Geometry check sheet. Reference: the model listing, model coordinates, mm. Give positions to 0.01 mm unless a question says otherwise; leave off trailing zeros.
```python
from build123d import *

# Parameters (mm, degrees)
SKETCH_1_R          = 2.5
EXTRUDE_1_DEPTH     = 506.79
CUT_EXTRUDE_1_DEPTH = 508.341254196


with BuildPart() as part:
    # 草图1 → 凸台-拉伸1 (new body)
    with BuildSketch(Plane(origin=(0, 0, 0), x_dir=(1, 0, 0), z_dir=(0, 1, 0))):
        with BuildLine():
            Line((-10.811269129, -4.789644731), (-12.611269129, -4.789644731))
            Line((-12.611269129, -4.789644731), (-12.611269129, -10.189644731))
            ThreePointArc((-12.611269129, -10.189644731), (-12.171929301, -11.250304902), (-11.111269129, -11.689644731))
            Line((-11.111269129, -11.689644731), (-5.711269129, -11.689644731))
            Line((-5.711269129, -11.689644731), (-5.711269129, -9.889644731))
            Line((-5.711269129, -9.889644731), (-8.111269129, -9.889644731))
            Line((-8.111269129, -9.889644731), (-8.111269129, -8.086694886))
            Line((-8.111269129, -8.086694886), (-4.814218974, -4.789644731))
            Line((-4.814218974, -4.789644731), (-0.408319284, -4.789644731))
            Line((-0.408319284, -4.789644731), (2.888730871, -8.086694886))
            Line((2.888730871, -8.086694886), (2.888730871, -9.889644731))
            Line((2.888730871, -9.889644731), (0.488730871, -9.889644731))
            Line((0.488730871, -9.889644731), (0.488730871, -11.689644731))
            Line((0.488730871, -11.689644731), (5.888730871, -11.689644731))
            ThreePointArc((5.888730871, -11.689644731), (6.949391043, -11.250304902), (7.388730871, -10.189644731))
            Line((7.388730871, -10.189644731), (7.388730871, -4.789644731))
            Line((7.388730871, -4.789644731), (5.588730871, -4.789644731))
            Line((5.588730871, -4.789644731), (5.588730871, -7.189644731))
            Line((5.588730871, -7.189644731), (3.785781026, -7.189644731))
            Line((3.785781026, -7.189644731), (0.442857891, -3.846721596))
            Line((0.442857891, -3.846721596), (0.442857891, 0.467432135))
            Line((0.442857891, 0.467432135), (3.785781026, 3.810355269))
            Line((3.785781026, 3.810355269), (5.588730871, 3.810355269))
            Line((5.588730871, 3.810355269), (5.588730871, 1.410355269))
            Line((5.588730871, 1.410355269), (7.388730871, 1.410355269))
            Line((7.388730871, 1.410355269), (7.388730871, 6.810355269))
            ThreePointArc((7.388730871, 6.810355269), (6.949391043, 7.871015441), (5.888730871, 8.310355269))
            Line((5.888730871, 8.310355269), (0.488730871, 8.310355269))
            Line((0.488730871, 8.310355269), (0.488730871, 6.510355269))
            Line((0.488730871, 6.510355269), (2.888730871, 6.510355269))
            Line((2.888730871, 6.510355269), (2.888730871, 4.707405425))
            Line((2.888730871, 4.707405425), (-0.408319284, 1.410355269))
            Line((-0.408319284, 1.410355269), (-4.814218974, 1.410355269))
            Line((-4.814218974, 1.410355269), (-8.111269129, 4.707405425))
            Line((-8.111269129, 4.707405425), (-8.111269129, 6.510355269))
            Line((-8.111269129, 6.510355269), (-5.711269129, 6.510355269))
            Line((-5.711269129, 6.510355269), (-5.711269129, 8.310355269))
            Line((-5.711269129, 8.310355269), (-11.111269129, 8.310355269))
            ThreePointArc((-11.111269129, 8.310355269), (-12.171929301, 7.871015441), (-12.611269129, 6.810355269))
            Line((-12.611269129, 6.810355269), (-12.611269129, 1.410355269))
            Line((-12.611269129, 1.410355269), (-10.811269129, 1.410355269))
            Line((-10.811269129, 1.410355269), (-10.811269129, 3.810355269))
            Line((-10.811269129, 3.810355269), (-9.008319284, 3.810355269))
            Line((-9.008319284, 3.810355269), (-5.665396149, 0.467432135))
            Line((-5.665396149, 0.467432135), (-5.665396149, -3.846721596))
            Line((-5.665396149, -3.846721596), (-9.008319284, -7.189644731))
            Line((-9.008319284, -7.189644731), (-10.811269129, -7.189644731))
            Line((-10.811269129, -7.189644731), (-10.811269129, -4.789644731))
        make_face()
        with Locations(Location((-2.611269129, -1.689644731, 0), (0, 0, 270))):
            Circle(SKETCH_1_R, mode=Mode.SUBTRACT)
    extrude(amount=EXTRUDE_1_DEPTH)

    # 草图2 → 切除-拉伸1 (cut, through all)
    with BuildSketch(Plane(origin=(0, 0, -8.310355269), x_dir=(-1, 0, 0), z_dir=(0, 0, -1))):
        Polygon((-7.388730871, 506.79), (12.611269129, 486.79), (12.611269129, 506.79), align=None)
        Polygon((12.611269129, 0), (-7.388730871, 20), (-7.388730871, 0), align=None)
    extrude(amount=-CUT_EXTRUDE_1_DEPTH, mode=Mode.SUBTRACT)


solid = part.part
```
Q1. Thickness scan on L1, parallel to X at y = 403.5, z = -7; L2, parallel to X at y = 229, z = 1; L3, parallel to X at y = 73, z = -3.5. Record the ranges inside material, lowest first.
Q2. Gauge pin test, flat ends, axial feed: P1, Ø10, axis at x = -1.5, z = -1, coming from the -Y side; P2, Ø6, axis at x = -2.61, z = 1.69, coming from the +Y side; P3, Ø3.5, axis at y = 261.5, z = 1.5, coming from the +X side. Record the tip position at first contact, or that the pin passes through.
Q3. Release check for a two-part mould opening along Y. For faces 1 (the face through (-4.97, 7.64, 3.77)), 2 (the face through (-4.7, 494.7, 3.8)) record: pulls with the +Y half, pulls with the -Y half, needs draft (parallel to the pull), parting line crosses it, or undercut.
Answers follow:
1. L1: x = -12.6 to -5.71, 0.49 to 7.38
1. L2: x = -5.67 to -5.01, -0.21 to 0.44
1. L3: x = -12.61 to -10.81, -8.7 to -6.9, 1.68 to 3.48, 5.59 to 7.39
2. P1: stops at y = 6.12
2. P2: stops at y = 499.79
2. P3: stops at x = 0.44
3. face 1: pulls with the -Y half
3. face 2: pulls with the +Y half
